Autodesk Inventor part; units mm, degrees
ref_plane "YZ Plane" through (0, 0, 0) normal (1, 0, 0) x (0, 1, 0)
ref_plane "XZ Plane" through (0, 0, 0) normal (0, 1, 0) x (-1, 0, 0)
ref_plane "XY Plane" through (0, 0, 0) normal (0, 0, 1) x (1, 0, 0)
sketch "Skizze2" plane through (0, 0, 0) normal (0, 1, 0) x (-1, 0, 0)
  line L0 (0, -6) -> (-14.85, -6)
  line L1 (-14.85, -6) -> (-14.85, -2.3274)
  line L2 (-14.85, -2.3274) -> (-13.85, -1.75)
  line L3 (-13.85, -1.75) -> (-13.85, 1.75)
  line L4 (-13.85, 1.75) -> (-14.85, 2.3274)
  line L5 (-14.85, 2.3274) -> (-14.85, 6)
  line L6 (-14.85, 6) -> (0, 6)
  line L7 (0, 6) -> (0, -6)
  point P0 (0, 0)
  point P1 (-13.85, 0)
  point P2 (0, 0)
  dimension "d3" = 29.7
  dimension "d4" = 12
  dimension "d5" = 3.5
  dimension "d6" = 120
  dimension "d7" = 120
  dimension "d8" = 1
revolve "Umdrehung1" add sketch "Skizze2" angle 360 about axis through (0, 0, 6) along (0, 0, -1)
sketch "Skizze3" plane through (0, 0, 6) normal (0, 0, 1) x (1, 0, 0)
  line L0 (-10, -3.75) -> (10, -3.75)
  line L1 (10, -3.75) -> (10, 3.75)
  line L2 (10, 3.75) -> (-10, 3.75)
  line L3 (-10, 3.75) -> (-10, -3.75)
  line L4 (-10, -3.75) -> (10, 3.75) construction
  line L5 (10, -3.75) -> (-10, 3.75) construction
  point P0 (0, 0)
  point P1 (0, 0)
  dimension "d10" = 20
  dimension "d11" = 7.5
  dimension "d12" = 0
extrude "Extrusion2" cut sketch "Skizze3" against normal through all
sketch "Skizze4" plane through (0, 0, -6) normal (0, 0, -1) x (-1, 0, 0)
  line L0 (-11.5, -1.8) -> (11.5, -1.8)
  line L1 (11.5, -1.8) -> (11.5, 0)
  line L2 (11.5, 0) -> (-11.5, 0)
  line L3 (-11.5, 0) -> (-11.5, -1.8)
  line L4 (-11.5, -1.8) -> (11.5, 0) construction
  line L5 (11.5, -1.8) -> (-11.5, 0) construction
  circle A0 centre (0, 0) radius 14.85
  point P0 (0, -0.9)
  dimension "d15" = 23
  dimension "d16" = 1.8
extrude "Extrusion3" cut sketch "Skizze4" against normal blind 10 contours L3 L2 L1 L0
fillet "Rundung1" radius 0.2 4 edges at (10, -3.75, 0) (-10, -3.75, 0) (-10, 3.75, 0) (10, 3.75, 0)
fillet "Rundung2" radius 0.2 8 edges at (-10, -1.8, -1) (-11.5, -1.8, -1) (-11.5, 0, -1) (-10, 0, -1) (10, -1.8, -1) (11.5, -1.8, -1) (11.5, 0, -1) (10, 0, -1)
properties part number "FMR_DXWD80_CPW_Halter_C_TdOS_Waveguide"
For this review, take the finished solid that the model builds, in its own axes (mm). A direction names the side the tool comes from. Round coordinates to 2 decimals unless told otherwise and drop trailing zeros. Write each loop counter-clockwise with the first axis right and the second up, starting at its lowest first coordinate (ties: lowest second). Pieces come first, ordered by that corner, then holes. Notation, with made-up numbers: (31, -9) - (61, -9) arc R13 ccw to (61, 12) - close; hole circle Ø4 at (-0.5, 16). An arc over 180 degrees is marked (long way). Use CSV: the item, a comma, the result in double quotes.
1) Clearance check with flat-ended pins moving along their axes: pin 1 Ø1 at (x, z) = (-1, -2) entering from +Y; pin 2 Ø1.2 at (x, z) = (11, 1) entering from -Y; pin 3 Ø0.9 at (x, z) = (-11, -2) entering from +Y. State where each tip first meets the part, or that it passes through.
Conclusion:
pin 1,"stops at y = 14.84"
pin 2,"stops at y = -9.15"
pin 3,"stops at y = 10.31"
2) For faces 1 (the flat face through (0, 6, 6)), 2 (the flat face through (11, -1.8, -1)), 3 (the flat face through (10, 1, 0)), 4 (the cylindrical face through (13.21, 4.16, 0.02)), list the 3-axis set-ups (+Z, -Z, +X, -X, +Y, -Y) from which the entire face can be reached by the end or side of a thin tool; tool diameter is ignored.
Conclusion:
face 1,"+Z, +X, -X, +Y, -Y"
face 2,"-Z"
face 3,"+Z, -Z"
face 4,"none"
3) Add section A-A on z = 5. Write out the cut boundary in (x, y).
Conclusion:
outline,"circle Ø29.7 at (0, 0); hole (-10, -3.55) arc R0.2 ccw to (-9.8, -3.75) - (9.8, -3.75) arc R0.2 ccw to (10, -3.55) - (10, 3.55) arc R0.2 ccw to (9.8, 3.75) - (-9.8, 3.75) arc R0.2 ccw to (-10, 3.55) - close"
4) Add section B-B on x = 0. Write out the cut boundary in (y, z).
Conclusion:
outline,"(-14.85, -6) - (-3.75, -6) - (-3.75, 6) - (-14.85, 6) - (-14.85, 2.33) - (-13.85, 1.75) - (-13.85, -1.75) - (-14.85, -2.33) - close; (3.75, -6) - (14.85, -6) - (14.85, -2.33) - (13.85, -1.75) - (13.85, 1.75) - (14.85, 2.33) - (14.85, 6) - (3.75, 6) - close"
5) Wall thickness on line 1 along Y through (x, z) = (0.25, -4); line 2 along Y through (x, z) = (-6, 0.5); line 3 along X through (y, z) = (-3.25, 5.75): over which ranges is each line inside the solid? List them lowest first. Write a range as from..to.
Conclusion:
line 1,"y = -14.85..-3.75, 3.75..14.85"
line 2,"y = -12.48..-3.75, 3.75..12.48"
line 3,"x = -14.49..-10, 10..14.49"
6) The part is to be moulded in two halves that separate along Y. For faces 5 (the flat face through (0, 6, -6)), 6 (the flat face through (11, -1, 4)), 7 (the cylindrical face through (-11.78, -9.04, -4.14)), say which applies: pulls with the +Y half, pulls with the -Y half, needs draft (parallel to the pull), parting line crosses it, or undercut.
Conclusion:
face 5,"needs draft"
face 6,"undercut"
face 7,"parting line crosses it"
